Design review of the part built by this model. Coordinates are the model's own, in mm. Face numbers are marked on the shaded views. A direction names the side the tool comes from. Round coordinates to 2 decimals unless told otherwise and drop trailing zeros. Order: outer loops, then holes, each group sorted by start corner. A loop starts at its lowest first (then second) coordinate and runs counter-clockwise, first axis right, second up. Notation, with made-up numbers: M -30,-33 L -11,-33 A33 cw -11,-2 Z; hole C 45,6 d10. An arc over 180 degrees is marked long. Use a Markdown table: item, result. Add a question column.
(1) Take a section at D-D (x = -9). Write out the cut boundary in (y, z), then the cut area to 3 significant figures.
(2) Machinability: for the marked faces 1 and 2, which of the approach directions +Z, -Z, +X, -X, +Y, -Y give a long, thin tool a straight path to every point of the face, cutting with its end or side? Answer none if there is none.
(3) Take a section at A-A (z = -10). Count the separate pieces of the cut face and the enclosed holes in it, then the cut area to 3 significant figures.
(4) For pin 1 (4 mm diameter, centred on x = -24.5, y = 11, fed in from +Z); pin 2 (8 mm diameter, centred on x = 14, z = -5.5, fed in from +Y); pin 3 (1.8 mm diameter, centred on x = -24.5, y = 11, fed in from +Z), all flat-tipped, find the tip position at first contact; note any pin that passes through.
(5) The part is to be moulded in two halves that separate along X. For the marked faces 3, 4, 5 and 6, say which applies: released by +X, released by -X, zero draft, split by the parting line, or undercut.
(6) Take a section at C-C (z = 0). Write out the cut boundary in (x, y), then the cut area to 3 significant figures.
(7) To check wall thickness, follow probe 1 along X at (y, z) = (1.45, 0); probe 2 along Y at (x, z) = (-24, -12.3); probe 3 along Z at (x, y) = (0, 1.5). State the ranges of each line that lie inside material, in increasing order. Write a range as from..to.
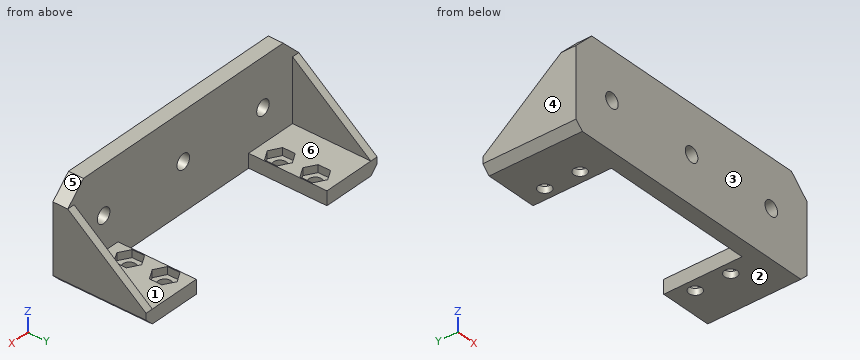
```python
from build123d import *

# Parameters (mm, degrees)
SKETCH1_W           = 73.66
SKETCH1_H           = 25.4
BOSS_EXTRUDE1_DEPTH = 4
CHAMFER1_SIZE       = 5
SKETCH2_R           = 2
SKETCH2_W           = 16
SKETCH2_H           = 3.728527123
BOSS_EXTRUDE2_DEPTH = 21
CUT_EXTRUDE1_START  = -31
SKETCH3_R           = 2
CUT_EXTRUDE1_DEPTH  = 31
BOSS_EXTRUDE3_DEPTH = 2
BOSS_EXTRUDE4_DEPTH = 2
CHAMFER2_SIZE       = 2
SKETCH7_R           = 1.7
CUT_EXTRUDE2_DEPTH  = 12
CUT_EXTRUDE3_DEPTH  = 2


with BuildPart() as part:
    # Sketch1 → Boss-Extrude1 (new body)
    with BuildSketch(Plane(origin=(0, 0, 0), x_dir=(1, 0, 0), z_dir=(0, 1, 0))):
        Rectangle(SKETCH1_W, SKETCH1_H)
    extrude(amount=BOSS_EXTRUDE1_DEPTH)

    # Chamfer1
    chamfer1_edges = [part.edges().sort_by_distance(p)[0] for p in [
        (36.83, 2, 12.7),
        (-36.83, 2, 12.7),
    ]]
    chamfer(chamfer1_edges, length=CHAMFER1_SIZE)

    # Sketch2 → Boss-Extrude2 (add)
    with BuildSketch(Plane(origin=(0, 4, 0), x_dir=(1, 0, 0), z_dir=(0, 1, 0))):
        with Locations(Location((-25.4, 0, 0), (0, 0, 90))):
            Circle(SKETCH2_R)
        with Locations(Location((0, 0, 0), (0, 0, 90))):
            Circle(SKETCH2_R)
        with Locations(Location((25.4, 0, 0), (0, 0, 90))):
            Circle(SKETCH2_R)
        with Locations((-28.83, 10.835736438)):
            Rectangle(SKETCH2_W, SKETCH2_H)
        with Locations((28.83, 10.835736438)):
            Rectangle(SKETCH2_W, SKETCH2_H)
    extrude(amount=BOSS_EXTRUDE2_DEPTH)

    # Sketch3 → Cut-Extrude1 (cut)
    with BuildSketch(Plane(origin=(0, 25, 0), x_dir=(1, 0, 0), z_dir=(0, 1, 0)).offset(CUT_EXTRUDE1_START)):
        with Locations(Location((-25.4, 0, 0), (0, 0, 270))):
            Circle(SKETCH3_R)
        with Locations(Location((0, 0, 0), (0, 0, 270))):
            Circle(SKETCH3_R)
        with Locations(Location((25.4, 0, 0), (0, 0, 270))):
            Circle(SKETCH3_R)
    extrude(amount=CUT_EXTRUDE1_DEPTH, mode=Mode.SUBTRACT)

    # Sketch4 → Boss-Extrude3 (add)
    with BuildSketch(Plane(origin=(36.83, 0, 0), x_dir=(0, 0, -1), z_dir=(1, 0, 0))):
        Polygon((8.971472877, 25), (-7.7, 4), (8.971472877, 4), align=None)
    extrude(amount=-BOSS_EXTRUDE3_DEPTH)

    # Sketch5 → Boss-Extrude4 (add)
    with BuildSketch(Plane.ZY.offset(36.83)):
        Polygon((-8.971472877, 25), (7.7, 4), (-8.971472877, 4), align=None)
    extrude(amount=-BOSS_EXTRUDE4_DEPTH)

    # Chamfer2
    chamfer2_edges = [part.edges().sort_by_distance(p)[0] for p in [
        (-36.83, 12.5, -12.7),
        (36.83, 12.5, -12.7),
    ]]
    chamfer(chamfer2_edges, length=CHAMFER2_SIZE)

    # Sketch7 → Cut-Extrude2 (cut)
    with BuildSketch(Plane.XY.offset(-8.971472877)):
        with Locations((-24, 19.2)):
            Circle(SKETCH7_R)
        with Locations((-24, 9.7)):
            Circle(SKETCH7_R)
        with Locations((24, 19.2)):
            Circle(SKETCH7_R)
        with Locations((24, 9.7)):
            Circle(SKETCH7_R)
    extrude(amount=-CUT_EXTRUDE2_DEPTH, mode=Mode.SUBTRACT)

    # Sketch8 → Cut-Extrude3 (cut)
    with BuildSketch(Plane.XY.offset(-8.971472877)):
        Polygon((-21.1, 17.525684219), (-21.1, 20.874315781), (-24, 22.548631561), (-26.9, 20.874315781), (-26.9, 17.525684219), (-24, 15.851368439), align=None)
        Polygon((-21.1, 11.4), (-24.022243186, 13.061473671), (-26.922243186, 11.361473671), (-26.9, 8), (-23.977756814, 6.338526329), (-21.077756814, 8.038526329), align=None)
        Polygon((21.1, 20.874315781), (21.1, 17.525684219), (24, 15.851368439), (26.9, 17.525684219), (26.9, 20.874315781), (24, 22.548631561), align=None)
        Polygon((21.1, 11.374315781), (21.1, 8.025684219), (24, 6.351368439), (26.9, 8.025684219), (26.9, 11.374315781), (24, 13.048631561), align=None)
    extrude(amount=-CUT_EXTRUDE3_DEPTH, mode=Mode.SUBTRACT)


solid = part.part
```
Verdict:
| question | item | result |
|---|---|---|
| 1 | outline | M 0,-12.7 L 4,-12.7 L 4,12.7 L 0,12.7 Z |
| 1 | area | 102 mm^2 |
| 2 | face 1 | +Z, +Y |
| 2 | face 2 | -Z, +X, -X, +Y, -Y |
| 3 | separate pieces | 1 |
| 3 | enclosed holes | 4 |
| 3 | area | 850 mm^2 |
| 4 | pin 1 | stops at z = -8.97 |
| 4 | pin 2 | stops at y = 4 |
| 4 | pin 3 | stops at z = -10.97 |
| 5 | face 3 | zero draft |
| 5 | face 4 | released by -X |
| 5 | face 5 | released by +X |
| 5 | face 6 | undercut |
| 6 | outline | M -36.83,0 L -27.4,0 L -27.4,4 L -34.83,4 L -34.83,13.7 L -36.83,13.7 Z; M -23.4,0 L -2,0 L -2,4 L -23.4,4 Z; M 2,0 L 23.4,0 L 23.4,4 L 2,4 Z; M 27.4,0 L 36.83,0 L 36.83,13.7 L 34.83,13.7 L 34.83,4 L 27.4,4 Z |
| 6 | area | 285 mm^2 |
| 7 | probe 1 | x = -36.83..-27.4, -23.4..-2, 2..23.4, 27.4..36.83 |
| 7 | probe 2 | y = 0..8, 11.4..17.5, 20.9..25 |
| 7 | probe 3 | z = -12.7..-2, 2..12.7 |
